from build123d import *

# Parameters (mm, degrees)
SKETCH1_W           = 174.17
SKETCH1_H           = 83
BOSS_EXTRUDE1_DEPTH = 7
SKETCH2_R           = 1.75
CUT_EXTRUDE1_DEPTH  = 8
SKETCH3_R           = 1.75
CUT_EXTRUDE2_DEPTH  = 8
SKETCH4_W           = 15.4
SKETCH4_H           = 10.4
SKETCH4_W_2         = 10.4
SKETCH4_H_2         = 15.4
CUT_EXTRUDE3_DEPTH  = 5
SKETCH5_W           = 10.4
SKETCH5_H           = 10.4
CUT_EXTRUDE4_DEPTH  = 5
SKETCH6_R           = 1.75
CUT_EXTRUDE5_DEPTH  = 3
SKETCH12_R          = 1.75
CUT_EXTRUDE9_DEPTH  = 8
CUT_EXTRUDE6_DEPTH  = 3.64
SKETCH9_W           = 10.4
SKETCH9_H           = 10.4
CUT_EXTRUDE7_DEPTH  = 5
SKETCH10_R          = 1.75
CUT_EXTRUDE8_DEPTH  = 3


with BuildPart() as part:
    # Sketch1 → Boss-Extrude1 (new body)
    with BuildSketch(Plane(origin=(0, 0, 0), x_dir=(1, 0, 0), z_dir=(0, 1, 0))):
        with Locations((87.085, 41.5)):
            Rectangle(SKETCH1_W, SKETCH1_H)
    extrude(amount=BOSS_EXTRUDE1_DEPTH)

    # Sketch2 → Cut-Extrude1 (cut, through all)
    with BuildSketch(Plane(origin=(0, 7, 0), x_dir=(1, 0, 0), z_dir=(0, 1, 0))):
        with Locations((87.085, 49.5)):
            Circle(SKETCH2_R)
        with Locations((77.585, 41.5)):
            Circle(SKETCH2_R)
        with Locations((96.585, 41.5)):
            Circle(SKETCH2_R)
        with Locations((87.085, 33.5)):
            Circle(SKETCH2_R)
    extrude(amount=-CUT_EXTRUDE1_DEPTH, mode=Mode.SUBTRACT)

    # Sketch3 → Cut-Extrude2 (cut, through all)
    with BuildSketch(Plane(origin=(0, 7, 0), x_dir=(1, 0, 0), z_dir=(0, 1, 0))):
        with Locations((87.085, 78)):
            Circle(SKETCH3_R)
        with Locations((5, 41.5)):
            Circle(SKETCH3_R)
        with Locations((87.085, 5)):
            Circle(SKETCH3_R)
        with Locations((169.17, 41.5)):
            Circle(SKETCH3_R)
    extrude(amount=-CUT_EXTRUDE2_DEPTH, mode=Mode.SUBTRACT)

    # Sketch4 → Cut-Extrude3 (cut)
    with BuildSketch(Plane(origin=(0, 7, 0), x_dir=(1, 0, 0), z_dir=(0, 1, 0))):
        with Locations((7.5, 41.5)):
            Rectangle(SKETCH4_W, SKETCH4_H)
        with Locations((87.085, 7.5)):
            Rectangle(SKETCH4_W_2, SKETCH4_H_2)
        with Locations((87.085, 75.5)):
            Rectangle(SKETCH4_W_2, SKETCH4_H_2)
        with Locations((166.67, 41.5)):
            Rectangle(SKETCH4_W, SKETCH4_H)
    extrude(amount=-CUT_EXTRUDE3_DEPTH, mode=Mode.SUBTRACT)

    # Sketch5 → Cut-Extrude4 (cut)
    with BuildSketch(Plane(origin=(0, 7, 0), x_dir=(1, 0, 0), z_dir=(0, 1, 0))):
        with Locations((74.585, 5)):
            Rectangle(SKETCH5_W, SKETCH5_H)
        with Locations((99.585, 5)):
            Rectangle(SKETCH5_W, SKETCH5_H)
    extrude(amount=-CUT_EXTRUDE4_DEPTH, mode=Mode.SUBTRACT)

    # Sketch6 → Cut-Extrude5 (cut, through all)
    with BuildSketch(Plane(origin=(0, 2, 0), x_dir=(1, 0, 0), z_dir=(0, 1, 0))):
        with Locations((74.585, 5)):
            Circle(SKETCH6_R)
        with Locations((99.585, 5)):
            Circle(SKETCH6_R)
    extrude(amount=-CUT_EXTRUDE5_DEPTH, mode=Mode.SUBTRACT)

    # Sketch12 → Cut-Extrude9 (cut, through all)
    with BuildSketch(Plane.XZ):
        with Locations((122.51393219, -26.25)):
            Circle(SKETCH12_R)
        with Locations((153.01393219, -26.25)):
            Circle(SKETCH12_R)
        with Locations((122.51393219, -56.75)):
            Circle(SKETCH12_R)
        with Locations((153.01393219, -56.75)):
            Circle(SKETCH12_R)
    extrude(amount=-CUT_EXTRUDE9_DEPTH, mode=Mode.SUBTRACT)

    # Sketch7 → Cut-Extrude6 (cut)
    with BuildSketch(Plane(origin=(0, 7, 0), x_dir=(1, 0, 0), z_dir=(0, 1, 0))):
        Polygon((75.824081679, 44.55), (79.345918321, 44.55), (81.106836642, 41.5), (79.345918321, 38.45), (75.824081679, 38.45), (74.063163358, 41.5), align=None)
        Polygon((85.324081679, 52.55), (88.845918321, 52.55), (90.606836642, 49.5), (88.845918321, 46.45), (85.324081679, 46.45), (83.563163358, 49.5), align=None)
        Polygon((100.106836642, 41.5), (98.345918321, 44.55), (94.824081679, 44.55), (93.063163358, 41.5), (94.824081679, 38.45), (98.345918321, 38.45), align=None)
        Polygon((83.563163358, 33.5), (85.324081679, 30.45), (88.845918321, 30.45), (90.606836642, 33.5), (88.845918321, 36.55), (85.324081679, 36.55), align=None)
        Polygon((120.753013869, 29.3), (124.274850511, 29.3), (126.035768832, 26.25), (124.274850511, 23.2), (120.753013869, 23.2), (118.992095548, 26.25), align=None)
        Polygon((151.253013869, 29.3), (154.774850511, 29.3), (156.535768832, 26.25), (154.774850511, 23.2), (151.253013869, 23.2), (149.492095548, 26.25), align=None)
        Polygon((151.253013869, 59.8), (154.774850511, 59.8), (156.535768832, 56.75), (154.774850511, 53.7), (151.253013869, 53.7), (149.492095548, 56.75), align=None)
        Polygon((120.753013869, 59.8), (124.274850511, 59.8), (126.035768832, 56.75), (124.274850511, 53.7), (120.753013869, 53.7), (118.992095548, 56.75), align=None)
    extrude(amount=-CUT_EXTRUDE6_DEPTH, mode=Mode.SUBTRACT)

    # Sketch9 → Cut-Extrude7 (cut)
    with BuildSketch(Plane.XZ):
        with Locations((71.585, -78)):
            Rectangle(SKETCH9_W, SKETCH9_H)
        with Locations((102.585, -78)):
            Rectangle(SKETCH9_W, SKETCH9_H)
    extrude(amount=-CUT_EXTRUDE7_DEPTH, mode=Mode.SUBTRACT)

    # Sketch10 → Cut-Extrude8 (cut, through all)
    with BuildSketch(Plane.XZ.offset(-5)):
        with Locations((71.585, -78)):
            Circle(SKETCH10_R)
        with Locations((102.585, -78)):
            Circle(SKETCH10_R)
    extrude(amount=-CUT_EXTRUDE8_DEPTH, mode=Mode.SUBTRACT)


solid = part.part
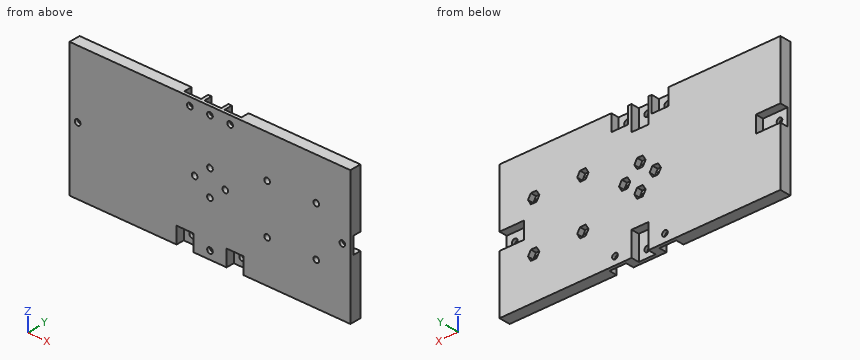
Source: CAD feature listing. Evaluate the final solid. Frame: model axes, mm. Round coordinates to 2 decimals unless told otherwise and drop trailing zeros. Loops run counter-clockwise (first coordinate to the right, second up) from the corner with the lowest first, then second, coordinate; pieces in that order, holes last. Notation, with made-up numbers: M 88.5,39 L 139.5,39 A26 ccw 139.5,60 Z; hole C 8.25,88.25 d6. An arc over 180 degrees is marked long. Return JSON: item names as keys, results as strings. Group by question number.
1. Section query B-B on z = -5. Output: boundary loops of the cut face in (x, y) (3 decimals), and give its area (3 significant figures).
2. Material intervals for line 1 along X through (y, z) = (0.75, -5) (3 decimals); line 2 along X through (y, z) = (6, -78) (3 decimals); line 3 along X through (y, z) = (5.25, -74) (3 decimals), sorted ascending. Write a range as from..to.
3. Section query C-C on x = 162. Output: boundary loops of the cut face in (y, z), and give its area (3 significant figures).
4. Section query A-A on x = 5. Output: boundary loops of the cut face in (y, z), and give its area (3 significant figures).
5. Pin query (flat end, axial travel): pin 1 (2.5 mm diameter, centred on x = 104, y = 2.5, fed in from -Z); pin 2 (4 mm diameter, centred on x = 153.01, z = -26.25, fed in from +Y); pin 3 (5 mm diameter, centred on x = 86.5, z = -4.5, fed in from +Y); pin 4 (2 mm diameter, centred on x = 122.51, z = -56.75, fed in from +Y). Return the tip coordinate at first contact, or that it passes through.
6. Section query D-D on z = -69.5. Output: boundary loops of the cut face in (x, y) (3 decimals), and give its area (3 significant figures).
Checks:
{
 "1": {"outline": "M 0,0 L 72.835,0 L 72.835,2 L 69.385,2 L 69.385,7 L 0,7 Z; M 76.335,0 L 85.335,0 L 85.335,2 L 81.885,2 L 81.885,7 L 79.785,7 L 79.785,2 L 76.335,2 Z; M 88.835,0 L 97.835,0 L 97.835,2 L 94.385,2 L 94.385,7 L 92.285,7 L 92.285,2 L 88.835,2 Z; M 101.335,0 L 174.17,0 L 174.17,7 L 104.785,7 L 104.785,2 L 101.335,2 Z", "area": "1,040 mm²"},
 "2": {"line 1": "x = 0..72.835, 76.335..85.335, 88.835..97.835, 101.335..174.17", "line 2": "x = 0..69.835, 73.335..81.885, 92.285..100.835, 104.335..174.17", "line 3": "x = 0..81.885, 92.285..174.17"},
 "3": {"outline": "M 0,-83 L 7,-83 L 7,-46.7 L 2,-46.7 L 2,-36.3 L 7,-36.3 L 7,0 L 0,0 Z", "area": "529 mm²"},
 "4": {"outline": "M 0,-83 L 7,-83 L 7,-46.7 L 2,-46.7 L 2,-43.25 L 0,-43.25 Z; M 0,-39.75 L 2,-39.75 L 2,-36.3 L 7,-36.3 L 7,0 L 0,0 Z", "area": "522 mm²"},
 "5": {"pin 1": "stops at z = -72.8", "pin 2": "stops at y = 3.36", "pin 3": "stops at y = 2", "pin 4": "passes through"},
 "6": {"outline": "M 0,0 L 174.17,0 L 174.17,7 L 92.285,7 L 92.285,2 L 81.885,2 L 81.885,7 L 0,7 Z", "area": "1,170 mm²"}
}
